Autodesk Inventor part; units mm, degrees
ref_plane "YZ Plane" through (0, 0, 0) normal (1, 0, 0) x (0, 1, 0)
ref_plane "XZ Plane" through (0, 0, 0) normal (0, 1, 0) x (-1, 0, 0)
ref_plane "XY Plane" through (0, 0, 0) normal (0, 0, 1) x (1, 0, 0)
sketch "Boceto1" plane through (0, 0, 0) normal (0, 1, 0) x (-1, 0, 0)
  circle A0 centre (20.1414, -70.1386) radius 1.5
  circle A1 centre (20.1414, -15.4215) radius 1.5
  line L0 (115.646, -75.4125) -> (-5.464, -75.4125)
  line L1 (20.1414, -75.4125) -> (15.1414, -75.4125)
  line L2 (15.1414, -75.4125) -> (25.1414, -75.4125)
  line L3 (25.1414, -75.4125) -> (25.1414, -10.4125)
  line L4 (25.1414, -10.4125) -> (15.1414, -10.4125)
  line L5 (15.1414, -10.4125) -> (15.1414, -75.4125)
  circle A2 centre (20.1414, -70.1386) radius 1.5
  circle A3 centre (20.1414, -15.4215) radius 1.5
  line L6 (115.646, -75.4125) -> (-5.464, -75.4125)
  line L7 (20.1414, -75.4125) -> (15.1414, -75.4125)
  line L8 (15.1414, -75.4125) -> (25.1414, -75.4125)
  line L9 (25.1414, -75.4125) -> (25.1414, -10.4125)
  line L10 (25.1414, -10.4125) -> (15.1414, -10.4125)
  line L11 (15.1414, -10.4125) -> (15.1414, -75.4125)
  point P0 (0, 0)
  dimension "d0" = 5
  dimension "d1" = 10
  dimension "d2" = 65
  dimension "d3" = 5
  dimension "d4" = 10
  dimension "d5" = 65
extrude "Extrusión1" add sketch "Boceto1" along normal blind 3
sketch "Boceto2" plane through (0, 3, 0) normal (0, 1, 0) x (1, 0, 0)
  line L0 (-15.1414, 75.4125) -> (-25.1414, 75.4125)
  line L1 (-15.1414, 10.4125) -> (-15.1414, 75.4125)
  line L2 (-25.1414, 75.4125) -> (-15.1414, 75.4125)
  line L3 (-15.1414, 75.4125) -> (-15.1414, 72.4125)
  line L4 (-15.1414, 72.4125) -> (-25.1414, 72.4125)
  line L5 (-25.1414, 72.4125) -> (-25.1414, 75.4125)
  point P0 (0, 0)
  dimension "d8" = 3
extrude "Extrusión2" add sketch "Boceto2" along normal blind 91
properties part number "piezasoportepantalla"
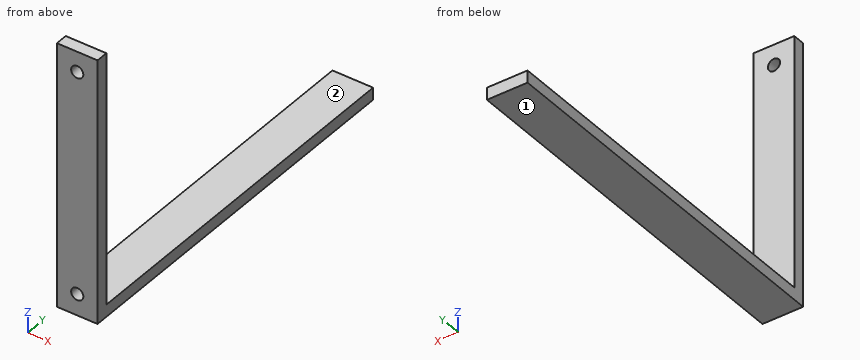
Read the model definition and answer for the solid it produces. Units are mm, in the model's axes. Face numbers are marked on the shaded views. A direction names the side the tool comes from. Coordinates: 2 decimals unless noted, no trailing zeros. Loops run counter-clockwise (first coordinate to the right, second up) from the corner with the lowest first, then second, coordinate; pieces in that order, holes last. Notation, with made-up numbers: (83.25, 59) - (116.25, 59) arc R12 ccw to (116.25, 78) - close; hole circle Ø11 at (-4.75, 23). An arc over 180 degrees is marked (long way). Answer in a Markdown table with one row per item.
1. Which of the six approach directions +Z, -Z, +X, -X, +Y, -Y give full straight-line access (tool end or side, diameter ignored) to the marked faces 1 and 2?
Conclusion:
| item | result |
|---|---|
| face 1 | -Z, +X, -X, +Y, -Y |
| face 2 | +Z, +X, -X, +Y |
2. Find section A-A, the plane x = -20.5. Write down the section's boundary in (y, z) (1 decimal), then the cut area to 3 significant figures.
Conclusion:
| item | result |
|---|---|
| outline | (0, -75.4) - (94, -75.4) - (94, -72.4) - (3, -72.4) - (3, -71.6) - (0, -71.6) - close; (0, -68.7) - (3, -68.7) - (3, -16.9) - (0, -16.9) - close; (0, -14) - (3, -14) - (3, -10.4) - (0, -10.4) - close |
| area | 451 mm² |
3. Find section C-C, the plane z = -42. Write down the section's boundary in (x, y), then the cut area to 3 significant figures.
Conclusion:
| item | result |
|---|---|
| outline | (-25.14, 0) - (-15.14, 0) - (-15.14, 3) - (-25.14, 3) - close |
| area | 30.0 mm² |
4. Find section B-B, the plane y = 33.5. Write down the section's boundary in (x, z).
Conclusion:
| item | result |
|---|---|
| outline | (-25.14, -75.41) - (-15.14, -75.41) - (-15.14, -72.41) - (-25.14, -72.41) - close |
5. Straight lines are drawn through the part: line 1 (Z direction, x = -23, y = 74); line 2 (Y direction, x = -15.75, z = -43.5). For each, find the intervals that lie inside material, in ascending order.
Conclusion:
| item | result |
|---|---|
| line 1 | z = -75.41 to -72.41 |
| line 2 | y = 0 to 3 |
6. Given pin 1 (4 mm diameter, centred on x = -20.14, z = -70.14, fed in from +Y); pin 2 (5 mm diameter, centred on x = -20.5, y = 46.5, fed in from +Z), each flat-ended and moving along its own axis, determine where each tip first touches the part or whether it passes through.
Conclusion:
| item | result |
|---|---|
| pin 1 | stops at y = 3 |
| pin 2 | stops at z = -72.41 |
